Here's how the part is built. I have some questions about the finished solid (model axes, mm). A direction names the side the tool comes from. Give positions to 0.01 mm unless a question says otherwise; leave off trailing zeros. Write each loop counter-clockwise with the first axis right and the second up, starting at its lowest first coordinate (ties: lowest second). Pieces come first, ordered by that corner, then holes. Notation, with made-up numbers: (61, 77) -> (100, 77) arc R21 cw to (100, 114) -> close; hole circle Ø8 at (58, -7.5). An arc over 180 degrees is marked (long way). Use CSV: the item, a comma, the result in double quotes. Start each with the question number.
(1) If we mould it in two halves opening along X, with no side actions, what happens to faces 1 (the cylindrical face through (95.2, 17.4, 2.5)), 2 (the cylindrical face through (58.263, 10.122, 11.403)), 3 (the flat face through (114.3, 19, 9)), 4 (the flat face through (43, 46.038, 12))? For each: pulls with the +X half, pulls with the -X half, needs draft (parallel to the pull), parting line crosses it, or undercut.
(2) Suppose I cut it at D-D on x = 95.25. List the corners of the cut face in (y, z) for me, plus the area to 3 significant figures.
(3) I need wall thicknesses on L1, parallel to Y at x = 59.95, z = 11.55; L2, parallel to Y at x = 59.95, z = 16.35; L3, parallel to X at y = 19, z = 1.75. Which ranges of each line are inside material? Lowest first, please. Write a range as [from, to].
(4) For pin 1 Ø4 at (x, y) = (30, 8) entering from +Z (3 decimals); pin 2 Ø2 at (y, z) = (42, 14) entering from +X; pin 3 Ø4 at (y, z) = (7, 16.5) entering from -X; pin 4 Ø6.5 at (x, y) = (28.95, 40.9) entering from -Z (3 decimals), each with a flat end and sliding along its axis, tell me the tip position at first contact or that it passes through.
(5) Suppose I cut it at A-A on x = 28.95. Give the number of separate pieces and of enclosed holes in the cut face, plus the area to 3 significant figures.
(6) Which directions (+Z, -Z, +X, -X, +Y, -Y) give clear straight access to the entire face, cutting with the end or side of a thin tool? Please do faces 5 (the flat face through (44, 41, 12.382)), 6 (the flat face through (22.86, 25, 5)), 7 (the flat face through (29, 8, 13.335)), 8 (the flat face through (85.09, 42, 10)).
(7) Suppose I cut it at B-B on y = 19.05. List the corners of the cut face in (x, z) for me (3 decimals), plus the area to 3 significant figures.
(8) Suppose I cut it at C-C on y = 13. List the corners of the cut face in (x, z) for me (3 decimals).
Autodesk Inventor part; units mm, degrees
ref_plane "YZ Plane" through (0, 0, 0) normal (1, 0, 0) x (0, 1, 0)
ref_plane "XZ Plane" through (0, 0, 0) normal (0, 1, 0) x (-1, 0, 0)
ref_plane "XY Plane" through (0, 0, 0) normal (0, 0, 1) x (1, 0, 0)
sketch "Sketch1" plane through (0, 0, 0) normal (0, 0, 1) x (1, 0, 0)
  line L0 (0, 0) -> (114.3, 0)
  line L1 (114.3, 0) -> (114.3, 46.0375)
  line L2 (114.3, 46.0375) -> (0, 46.0375)
  line L3 (0, 46.0375) -> (0, 0)
  line L4 (69.85, 46.0375) -> (19.05, 46.0375)
  point P0 (44.45, 46.0375)
  dimension "d0" = 114.3
  dimension "d1" = 46.0375
  dimension "d62" = 69.85
extrude "Extrusion1" add sketch "Sketch1" along normal blind 19.05
sketch "Sketch2" plane through (0, 0, 0) normal (0, 0, -1) x (-1, 0, 0)
  line L0 (-114.3, 46.0375) -> (0, 46.0375)
  line L1 (-114.3, 0) -> (-114.3, 46.0375)
  point P0 (0, 0)
  point P1 (-44.45, 25.4)
  point P2 (-19.05, 38.1)
  point P3 (0, 46.0375)
  dimension "d7" = 20.6375
  dimension "d8" = 69.85
hole "Hole1" at (44.45, 25.4, 0) direction (0, 0, 1) diameter 22 depth 25.4 tip angle 118
sketch "Sketch3" plane through (0, 0, 0) normal (0, 0, -1) x (-1, 0, 0)
  line L0 (-66.04, 3.81) -> (-22.86, 3.81)
  line L1 (-22.86, 3.81) -> (-22.86, 46.99)
  line L2 (-22.86, 46.99) -> (-66.04, 46.99)
  line L3 (-66.04, 46.99) -> (-66.04, 3.81)
  line L4 (-66.04, 3.81) -> (-22.86, 46.99) construction
  line L5 (-22.86, 3.81) -> (-66.04, 46.99) construction
  line L6 (-114.3, 46.0375) -> (0, 46.0375)
  line L7 (-69.85, 46.0375) -> (-19.05, 46.0375)
  line L8 (-66.04, 46.99) -> (-22.86, 46.99)
  line L9 (-22.86, 46.99) -> (-22.86, 46.0375)
  line L10 (-22.86, 46.0375) -> (-66.04, 46.0375)
  line L11 (-66.04, 46.0375) -> (-66.04, 46.99)
  line L12 (-114.3, 0) -> (-114.3, 46.0375)
  point P0 (0, 0)
  point P1 (-44.45, 25.4)
  point P2 (-19.05, 38.1)
  point P3 (0, 46.0375)
  dimension "d16" = 20.6375
  dimension "d17" = 43.18
  dimension "d18" = 43.18
  dimension "d21" = 69.85
  dimension "d22" = 43.18
extrude "Extrusion2" cut sketch "Sketch3" against normal blind 9.525
sketch "Sketch4" plane through (0, 0, 19.05) normal (0, 0, 1) x (1, 0, 0)
  line L0 (28.95, 9.9) -> (59.95, 9.9)
  line L1 (59.95, 9.9) -> (59.95, 40.9)
  line L2 (59.95, 40.9) -> (28.95, 40.9)
  line L3 (28.95, 40.9) -> (28.95, 9.9)
  line L4 (28.95, 9.9) -> (59.95, 40.9) construction
  line L5 (59.95, 9.9) -> (28.95, 40.9) construction
  line L6 (114.3, 46.0375) -> (0, 46.0375)
  line L7 (114.3, 0) -> (114.3, 46.0375)
  point P0 (0, 0)
  point P1 (44.45, 25.4)
  point P2 (69.85, 38.1)
  point P3 (0, 46.0375)
  dimension "d23" = 20.6375
  dimension "d24" = 69.85
  dimension "d25" = 31
  dimension "d26" = 31
hole "Hole2" at (28.95, 40.9, 19.05) at (28.95, 9.9, 19.05) at (59.95, 40.9, 19.05) at (59.95, 9.9, 19.05) direction (0, 0, -1) diameter 3.4036 end through all counterbore diameter 8.4074 counterbore depth 5.715
sketch "Sketch5" plane through (0, 0, 0) normal (0, -1, 0) x (1, 0, 0)
  line L0 (95.25, 9.525) -> (9.525, 9.525)
  line L1 (0, 0) -> (114.3, 0)
  line L2 (114.3, 0) -> (114.3, 19.05)
  dimension "d34" = 85.725
  dimension "d35" = 9.525
  dimension "d36" = 19.05
hole "Hole3" at (95.25, 0, 9.525) at (9.525, 0, 9.525) direction (0, 1, 0) diameter 9.6012 end through all
sketch "Sketch6" plane through (0, 0, 0) normal (0, 0, -1) x (-1, 0, 0)
  line L0 (-114.3, 46.0375) -> (0, 46.0375)
  line L1 (0, 46.0375) -> (0, 0)
  line L2 (0, 0) -> (-114.3, 0)
  line L3 (-100.0506, 46.0375) -> (-90.4494, 46.0375)
  line L4 (-114.3, 0) -> (-114.3, 46.0375)
  line L5 (-14.3256, 46.0375) -> (-4.7244, 46.0375)
  point P0 (-19.05, 38.1)
  point P1 (-95.25, 19.05)
  point P2 (-9.525, 19.05)
  point P3 (-19.05, 46.0375)
  point P4 (-22.86, 0)
  dimension "d105" = 19.05
  dimension "d108" = 19.05
  dimension "d110" = 9.6012
  dimension "d111" = 4.8006
  dimension "d112" = 9.525
hole "Hole4" at (95.25, 19.05, 0) at (9.525, 19.05, 0) direction (0, 0, 1) diameter 3.302 depth 12.2936 tip angle 118
sketch "Sketch8" plane through (114.3, 0, 0) normal (1, 0, 0) x (0, 0, -1)
  line L0 (-19.05, 46.0375) -> (-19.05, 0)
  line L1 (0, 0) -> (-19.05, 0)
  line L2 (0, 46.0375) -> (-19.05, 46.0375)
  point P0 (-9.525, 9.525)
  point P1 (-9.525, 28.575)
  dimension "d87" = 19.05
  dimension "d88" = 9.525
  dimension "d90" = 9.525
  dimension "d99" = 9.525
hole "Hole8" at (114.3, 9.525, 9.525) at (114.3, 28.575, 9.525) direction (-1, 0, 0) diameter 3.302 depth 12.2936 tip angle 118
sketch "Sketch11" plane through (0, 46.0375, 19.05) normal (0, 1, 0) x (1, 0, 0)
  line L0 (66.04, 9.525) -> (22.86, 9.525)
  line L1 (114.3, 0) -> (0, 0)
  line L2 (22.86, 9.525) -> (22.86, 19.05)
  line L3 (66.04, 19.05) -> (66.04, 9.525)
  point P0 (0, 19.05)
  point P1 (44.45, 4.7625)
  dimension "d114" = 9.525
  dimension "d115" = 43.18
  dimension "d116" = 4.7625
  dimension "d117" = 21.59
hole "Hole9" at (44.45, 46.0375, 14.2875) direction (0, -1, 0) diameter 3.81 depth 19.05 tip angle 118
sketch "Sketch14" plane through (0, 46.0375, 19.05) normal (0, 1, 0) x (1, 0, 0)
  line L0 (0, 0) -> (114.3, 0)
  line L1 (0, 19.05) -> (114.3, 19.05)
  line L2 (114.3, 0) -> (85.09, 0)
  line L3 (85.09, 0) -> (85.09, 19.05)
  line L4 (85.09, 19.05) -> (114.3, 19.05)
  line L5 (114.3, 19.05) -> (114.3, 0)
  dimension "d130" = 29.21
extrude "Extrusion5" cut sketch "Sketch14" against normal blind 7.9375
sketch "Sketch15" plane through (0, 0, 0) normal (0, 0, -1) x (-1, 0, 0)
  line L0 (-22.86, 3.81) -> (-66.04, 3.81)
  line L1 (-66.04, 3.81) -> (-66.04, 46.0375)
  line L2 (-85.09, 38.1) -> (-114.3, 38.1)
  line L3 (-85.09, 46.0375) -> (-85.09, 38.1)
  point P0 (0, 0)
  point P1 (-78.74, 15.875)
  point P2 (-85.09, 33.782)
  dimension "d133" = 12.065
  dimension "d134" = 12.7
  dimension "d135" = 4.318
  dimension "d136" = 0
hole "Hole10" at (78.74, 15.875, 0) at (85.09, 33.782, 0) direction (0, 0, 1) diameter 3.302 depth 12.2936 tip angle 118
sketch "Sketch16" plane through (0, 46.0375, 19.05) normal (0, 1, 0) x (1, 0, 0)
  point P0 (0, 19.05)
sketch "Sketch17" plane through (0, 46.0375, 19.05) normal (0, 1, 0) x (1, 0, 0)
  circle A0 centre (44.45, 4.7625) radius 1.905
  line L0 (0, 0) -> (114.3, 0)
  line L1 (44.45, 6.6675) -> (41.2634, 6.6675)
  line L2 (41.2634, 6.6675) -> (41.2634, 0)
  line L3 (41.2634, 0) -> (44.45, 0)
  line L4 (44.45, 0) -> (44.45, 6.6675)
  line L5 (44.45, 6.6675) -> (47.625, 6.6675)
  line L6 (47.625, 6.6675) -> (47.625, 0)
  line L7 (47.625, 0) -> (44.45, 0)
  line L8 (44.45, 0) -> (44.45, 6.6675)
  point P0 (0, 19.05)
  dimension "d144" = 3.175
extrude "Extrusion6" cut sketch "Sketch17" against normal blind 25.4
sketch "Sketch9" plane through (0, 0, 0) normal (0, 0, -1) x (-1, 0, 0)
  line L0 (-139.7, 41.275) -> (0, 41.275)
  line L1 (0, 0) -> (-114.3, 0)
  line L2 (-101.6, 31.369) -> (-38.1, 31.369)
  line L3 (0, 46.0375) -> (0, 0)
  line L4 (-19.05, 46.0375) -> (0, 46.0375)
  line L5 (0, 46.0375) -> (-31.75, 41.275)
  line L6 (-4.5219, 55.376) -> (-36.0166, 50.6518)
  point P0 (-19.05, 38.1)
  point P1 (-23.7267, 67.9523)
  dimension "d63" = 41.275
  dimension "d64" = 9.906
  dimension "d65" = 139.7
  dimension "d66" = 0
  dimension "d67" = 31.75
  dimension "d68" = 9.906
  dimension "d69" = 9.906
  dimension "d71" = 63.5
  dimension "d72" = 38.1
sketch "Sketch7" plane through (0, 0, 0) normal (-1, 0, 0) x (0, 0, 1)
  line L0 (9.525, 46.0375) -> (9.525, 3.81)
  line L1 (9.525, 24.9237) -> (9.525, -32.2263)
  point P0 (0, 0)
  point P1 (9.525, 89.85)
  dimension "d54" = 57.15
properties part number "ps system back mount"
Geometry says:
1,face 1,"undercut"
1,face 2,"undercut"
1,face 3,"pulls with the +X half"
1,face 4,"needs draft"
2,outline,"(0, 0) -> (17.4, 0) -> (17.4, 4.72) -> (0, 4.72) -> close; (0, 14.33) -> (38.1, 14.33) -> (38.1, 19.05) -> (0, 19.05) -> close; (20.7, 0) -> (38.1, 0) -> (38.1, 4.72) -> (20.7, 4.72) -> close"
2,area,"344 mm²"
3,L1,"[0, 8.2], [11.6, 39.2], [42.6, 46.04]"
3,L2,"[0, 5.7], [14.1, 36.7], [45.1, 46.04]"
3,L3,"[0, 7.87], [11.18, 22.86], [66.04, 93.6], [96.9, 114.3]"
4,pin 1,"z = 13.335"
4,pin 2,"x = 85.09"
4,pin 3,"x = 0"
4,pin 4,"z = 9.525"
5,separate pieces,"3"
5,enclosed holes,"0"
5,area,"353 mm²"
6,face 5,"+Z, +Y"
6,face 6,"-Z, +Y"
6,face 7,"+Z"
6,face 8,"+Z, -Z, +X, +Y"
7,outline,"(0, 0) -> (7.874, 0) -> (7.874, 5.017) arc R4.801 cw (long way) to (11.176, 5.017) -> (11.176, 0) -> (22.86, 0) -> (22.86, 9.525) -> (35.468, 9.525) -> (35.468, 19.05) -> (0, 19.05) -> close; (53.432, 9.525) -> (66.04, 9.525) -> (66.04, 0) -> (93.599, 0) -> (93.599, 5.017) arc R4.801 cw (long way) to (96.901, 5.017) -> (96.901, 0) -> (114.3, 0) -> (114.3, 19.05) -> (53.432, 19.05) -> close"
7,area,"1,420 mm²"
8,outline,"(0, 0) -> (22.86, 0) -> (22.86, 9.525) -> (66.04, 9.525) -> (66.04, 0) -> (114.3, 0) -> (114.3, 19.05) -> (62.789, 19.05) -> (62.789, 13.335) -> (57.111, 13.335) -> (57.111, 19.05) -> (31.789, 19.05) -> (31.789, 13.335) -> (26.111, 13.335) -> (26.111, 19.05) -> (0, 19.05) -> close; hole circle Ø9.601 at (9.525, 9.525); hole circle Ø9.601 at (95.25, 9.525)"
